Autodesk Inventor part; units mm, degrees
ref_plane "YZ Plane" through (0, 0, 0) normal (1, 0, 0) x (0, 1, 0)
ref_plane "XZ Plane" through (0, 0, 0) normal (0, 1, 0) x (-1, 0, 0)
ref_plane "XY Plane" through (0, 0, 0) normal (0, 0, 1) x (1, 0, 0)
sketch "Sketch1" plane through (0, 0, 0) normal (0, 0, 1) x (1, 0, 0)
  line L0 (0, 0) -> (25.4, 0)
  line L1 (25.4, 0) -> (25.4, 3.175)
  line L2 (3.175, 76.2) -> (0, 76.2)
  line L3 (0, 76.2) -> (0, 0)
  line L4 (3.175, 76.2) -> (3.175, 3.175)
  line L5 (3.175, 3.175) -> (25.4, 3.175)
  dimension "d0" = 3.175
  dimension "d1" = 3.175
  dimension "d2" = 76.2
  dimension "d3" = 25.4
extrude "Extrusion1" add sketch "Sketch1" along normal blind 25.4
sketch "Sketch2" plane through (0, 0, 0) normal (0, -1, 0) x (1, 0, 0)
  line L0 (25.4, 25.4) -> (0, 25.4)
  line L1 (0, 0) -> (25.4, 0)
  line L2 (25.4, 0) -> (25.4, 25.4)
  circle A0 centre (12.7, 19.05) radius 3.175
  circle A1 centre (12.7, 6.35) radius 3.175
  dimension "d6" = 12.7
  dimension "d7" = 6.35
  dimension "d8" = 6.35
  dimension "d9" = 6.35
  dimension "d10" = 6.35
  dimension "d11" = 12.7
extrude "Extrusion2" cut sketch "Sketch2" against normal blind 25.4
sketch "Sketch3" plane through (0, 0, 0) normal (-1, 0, 0) x (0, 0, 1)
  line L0 (25.4, 0) -> (25.4, 76.2)
  line L1 (0, 0) -> (25.4, 0)
  circle A0 centre (12.7, 57.912) radius 3.175
  line L2 (0, 76.2) -> (0, 0)
  arc A1 (25.4, 57.912) -> (0, 57.912) centre (12.7, 57.912) ccw
  line L3 (0, 76.2) -> (25.4, 76.2)
  line L4 (0, 57.912) -> (0, 76.2)
  line L5 (25.4, 76.2) -> (25.4, 57.912)
  line L6 (25.4, 76.2) -> (0, 76.2)
  dimension "d14" = 6.35
  dimension "d15" = 57.912
  dimension "d16" = 12.7
extrude "Extrusion3" cut sketch "Sketch3" against normal blind 25.4 contours A1 L2 L3 L0 | A0
equation "\"d1\" = d0"
equation "\"d10\" = d8"
equation "\"d11\" = d6"
properties part number "uptake support bracket"
Source: CAD feature listing. Evaluate the final solid. Frame: model axes, mm. A direction names the side the tool comes from. Round coordinates to 2 decimals unless told otherwise and drop trailing zeros. Loops run counter-clockwise (first coordinate to the right, second up) from the corner with the lowest first, then second, coordinate; pieces in that order, holes last.
(1) Section query C-C (z = 21.5). Output: boundary loops of the cut face in (x, y) (3 decimals).
From the geometry:
outline: (0, 0) - (10.681, 0) - (10.681, 3.175) - (3.175, 3.175) - (3.175, 67.069) - (0, 67.069) - close; (14.719, 0) - (25.4, 0) - (25.4, 3.175) - (14.719, 3.175) - close
(2) Section query D-D (x = 21.5). Output: boundary loops of the cut face in (y, z) (3 decimals), and give its area (3 significant figures).
From the geometry:
outline: (0, 0) - (3.175, 0) - (3.175, 25.4) - (0, 25.4) - close
area: 80.6 mm2
(3) Contact query for flat-ended pins moving along their axis: pin 1 Ø3 at (x, z) = (13, 16.5) entering from +Y (3 decimals); pin 2 Ø3 at (x, z) = (3, 4) entering from +Y. Output: stop coordinate, or through.
From the geometry:
pin 1: stops at y = 3.175
pin 2: stops at y = 68.37
(4) Pull-direction query (Y, two-part tool) for faces 1 (the flat face through (13, 0, 13)), 2 (the cylindrical face through (1.57, 61.06, 12.29)), 3 (the cylindrical face through (12.01, 1.57, 15.95)); classes: +Y half, -Y half, draft (parallel to the pull), parting line (faces both ways), or undercut.
From the geometry:
face 1: -Y half
face 2: undercut
face 3: draft
(5) Section query B-B (x = 12.7). Output: boundary loops of the cut face in (y, z) (3 decimals).
From the geometry:
outline: (0, 0) - (3.175, 0) - (3.175, 3.175) - (0, 3.175) - close; (0, 9.525) - (3.175, 9.525) - (3.175, 15.875) - (0, 15.875) - close; (0, 22.225) - (3.175, 22.225) - (3.175, 25.4) - (0, 25.4) - close
(6) Material intervals for probe 1 along Z at (x, y) = (12.7, 1.6) (3 decimals); probe 2 along X at (y, z) = (7.5, 8.25) (3 decimals); probe 3 along Y at (x, z) = (1.35, 12.7), sorted ascending.
From the geometry:
probe 1: z = 0 to 3.175, 9.525 to 15.875, 22.225 to 25.4
probe 2: x = 0 to 3.175
probe 3: y = 0 to 54.74, 61.09 to 70.61
(7) Section query A-A (z = 12.7). Output: boundary loops of the cut face in (x, y) (3 decimals), and give its area (3 significant figures).
From the geometry:
outline: (0, 0) - (25.4, 0) - (25.4, 3.175) - (3.175, 3.175) - (3.175, 54.737) - (0, 54.737) - close; (0, 61.087) - (3.175, 61.087) - (3.175, 70.612) - (0, 70.612) - close
area: 275 mm2
(8) Access query for faces 4 (the flat face through (3.175, 37, 13)), 5 (the flat face through (2, 23, 25.4)). Directions: +Z, -Z, +X, -X, +Y, -Y. A direction counts if a zero-diameter tool reaches every point of the face in a straight line with its end or side. Return the directions, or none.
From the geometry:
face 4: +Z, -Z, +X, +Y
face 5: +Z, +X, -X, +Y, -Y
